```python
from build123d import *


with BuildPart() as part:
    # Sketch2 → Revolve1 (revolve)
    with BuildSketch(Plane.XY, mode=Mode.PRIVATE) as revolve1_sk:
        with BuildLine():
            Line((-24.319148936, 9.525), (7.430851064, 9.525))
            Line((7.430851064, 9.525), (7.430851064, 15.875))
            Line((7.430851064, 15.875), (7.316402096, 15.875))
            ThreePointArc((7.316402096, 15.875), (-0.336356408, 18.650515004), (-4.430671947, 25.686478088))
            Line((-4.430671947, 25.686478088), (-13.222804096, 74.254906544))
            ThreePointArc((-13.222804096, 74.254906544), (-12.86536093, 75.607360219), (-11.59820875, 76.2))
            Line((-11.59820875, 76.2), (-2.094148936, 76.2))
            Line((-2.094148936, 76.2), (-2.094148936, 88.9))
            Line((-2.094148936, 88.9), (-24.319148936, 88.9))
            Line((-24.319148936, 88.9), (-24.319148936, 76.2))
            Line((-24.319148936, 76.2), (-23.449860757, 76.2))
            ThreePointArc((-23.449860757, 76.2), (-22.391500538, 75.81615218), (-21.82526541, 74.843093456))
            Line((-21.82526541, 74.843093456), (-11.692237493, 18.867451471))
            ThreePointArc((-11.692237493, 18.867451471), (-12.242150056, 16.78675351), (-14.191614948, 15.875))
            Line((-14.191614948, 15.875), (-24.319148936, 15.875))
            Line((-24.319148936, 15.875), (-24.319148936, 9.525))
        make_face()
    revolve(revolve1_sk.sketch.rotate(Axis((-25.028457447, 0, 0), (1, 0, 0)), 90), axis=Axis((-25.028457447, 0, 0), (1, 0, 0)))


solid = part.part
```
Input: part model. Units: mm. Frame: model coordinates. A direction names the side the tool comes from. Round coordinates to 2 decimals unless told otherwise and drop trailing zeros. Order: outer loops, then holes, each group sorted by start corner. A loop starts at its lowest first (then second) coordinate and runs counter-clockwise, first axis right, second up. Notation, with made-up numbers: (6, 58.25) - (42, 58.25) arc R24 ccw to (42, 82.25) - close; hole circle Ø1 at (78.5, -1.75). An arc over 180 degrees is marked (long way). One line per question, with ' | ' between items. Start each with the question number.
1) Ray query, probe 1 along Y at (x, z) = (-23.7, 0) (3 decimals); probe 2 along Y at (x, z) = (-6.5, 41.5); probe 3 along Y at (x, z) = (-3, -1.5). Return the intervals inside material, ascending.
2) Cut plane C-C, the plane x = -9. Return the cut outline in (y, z) (3 decimals).
3) Set-up query: faces 5 (the cylindrical face through (-6.78, 74.388, -16.519)), 6 (the flat face through (7.431, 7, -7)), 7 (the cylindrical face through (-23.878, 74.388, -16.519)). Return all of +Z, -Z, +X, -X, +Y, -Y with unobstructed straight access to the full face (end or side cutting, diameter ignored); none if empty.
4) Pull-direction query (Z, two-part tool) for faces 1 (the flat face through (-2.094, -39.9, -65.4)), 2 (the cylindrical face through (-13.362, -60.083, -65.523)), 3 (the conical face through (-12.184, -6.484, 20.589)), 4 (the cylindrical face through (-19.326, 15.497, -3.441)); classes: +Z half, -Z half, draft (parallel to the pull), parting line (faces both ways), or undercut.
5) Cut plane D-D, the plane x = 3. Return the cut outline in (y, z) (3 decimals), then the cut area to 3 significant figures.
6) Contact query for flat-ended pins moving along their axis: P1, Ø1.5, axis at x = 3, z = -8, coming from the -Y side; P2, Ø6, axis at x = -1.5, z = 47, coming from the +Y side; P3, Ø6, axis at x = -11, y = -37, coming from the -Z side; P4, Ø22, axis at y = 0, z = 0, coming from the +X side. Output: stop coordinate, or through.
Worked out:
1) probe 1: y = -88.9 to -76.2, -15.875 to -9.525, 9.525 to 15.875, 76.2 to 88.9 | probe 2: y = -78.62 to -63.91, 63.91 to 78.62 | probe 3: y = -88.89 to -76.19, -21.75 to -9.41, 9.41 to 21.75, 76.19 to 88.89
2) outline: circle Ø177.8 at (0, 0); circle Ø101.856 at (0, 0); hole circle Ø152.4 at (0, 0); hole circle Ø19.05 at (0, 0)
3) face 5: +X | face 6: +Z, -Z, +X, +Y, -Y | face 7: -X
4) face 1: draft | face 2: parting line | face 3: undercut | face 4: undercut
5) outline: circle Ø33.365 at (0, 0); hole circle Ø19.05 at (0, 0) | area: 589 mm^2
6) P1: stops at y = -15.16 | P2: stops at y = 77.21 | P3: stops at z = -82.14 | P4: stops at x = 7.43
